Source: CAD feature listing. Evaluate the final solid. Frame: model axes, mm. Face numbers are marked on the shaded views. A direction names the side the tool comes from. Round coordinates to 2 decimals unless told otherwise and drop trailing zeros. Order: outer loops, then holes, each group sorted by start corner. A loop starts at its lowest first (then second) coordinate and runs counter-clockwise, first axis right, second up. Notation, with made-up numbers: (7.25, -30.5) - (50.25, -30.5) arc R7 cw to (50.25, -22.5) - close; hole circle Ø3 at (-35.5, 15). An arc over 180 degrees is marked (long way). Return JSON: item names as keys, results as strings. Group by question number.
1) Section D-D, the plane y = 14. Return loops of the section in (x, z), plus the area to 3 significant figures.
2) Section B-B, the plane y = -11. Return loops of the section in (x, z), plus the area to 3 significant figures.
3) Mould query, pull axis X, two halves, no side actions, for the marked faces 1, 2, 3 and 4. Classes: pulls with the +X half, pulls with the -X half, needs draft (parallel to the pull), parting line crosses it, or undercut.
4) Section C-C, the plane x = 32. Return loops of the section in (y, z), plus the area to 3 significant figures.
5) Access query for the marked faces 5, 6, 7 and 8. Directions: +Z, -Z, +X, -X, +Y, -Y. A direction counts if a zero-diameter tool reaches every point of the face in a straight line with its end or side. Return the directions, or none.
6) Contact query for flat-ended pins moving along their axis: P1, Ø1.5, axis at y = 26.5, z = 3, coming from the +X side; P2, Ø1, axis at y = 24.5, z = 5, coming from the +X side; P3, Ø3, axis at x = 24.5, z = 8, coming from the +Y side. Output: stop coordinate, or through.
7) Ray query, line 1 (Y direction, x = 27, z = 7.5); line 2 (Z direction, x = 22, y = 8.5); line 3 (X direction, y = 14, z = 11.25). Return the intervals inside material, ascending. Write a range as from..to.
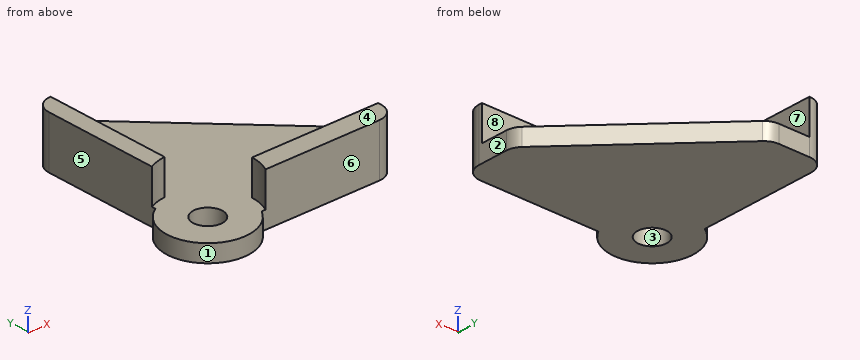
```python
from build123d import *

# Parameters (mm, degrees)
F1_R     = 4.25
F2_DEPTH = 5
F3_DEPTH = 15
F4_R     = 4.99999


# Not quite as in the source:
# - a fillet or chamfer is up to 0.001 mm smaller than in the source, because OpenCascade refuses the exact size
# - a feature names something its author has since deleted; it is built from what else it names


with BuildPart() as f2:
    # F1 (on Top) → F2 (new body)
    with BuildSketch(Plane.XY):
        with BuildLine():
            Line((39.3818591636, 0.8618591636), (-0.6181408364, 0.8618591636))
            Line((-0.6181408364, 0.8618591636), (-0.6181408364, 40.8618591636))
            Line((-0.6181408364, 40.8618591636), (-11.6181408364, 40.8618591636))
            Line((-11.6181408364, 40.8618591636), (-11.6181408364, 3.8233405604))
            ThreePointArc((-11.6181408364, 3.8233405604), (-14.1903183566, 3.3614410672), (-16.6181408364, 2.3944217582))
            Line((-16.6181408364, 2.3944217582), (-16.6181408364, 1.254164009))
            ThreePointArc((-16.6181408364, 1.254164009), (-19.1034222107, -17.6234222107), (-0.225835991, -15.1381408364))
            Line((-0.225835991, -15.1381408364), (0.9144217582, -15.1381408364))
            ThreePointArc((0.9144217582, -15.1381408364), (2.0096719934, -12.2265616521), (2.3818591636, -9.1381408364))
            Line((2.3818591636, -9.1381408364), (39.3818591636, -9.1381408364))
            Line((39.3818591636, -9.1381408364), (39.3818591636, 0.8618591636))
        make_face()
        with Locations((-10.6181408364, -9.1381408364)):
            Circle(F1_R, mode=Mode.SUBTRACT)
        Polygon((-0.6181408364, 40.8618591636), (-0.6181408364, 0.8618591636), (39.3818591636, 0.8618591636), align=None)
    extrude(amount=F2_DEPTH)

    # F1 (on Top) → F3 (join)
    with BuildSketch(Plane.XY):
        with BuildLine():
            Line((39.3818591636, -15.1381408364), (39.3818591636, -9.1381408364))
            Line((39.3818591636, -9.1381408364), (2.3818591636, -9.1381408364))
            ThreePointArc((2.3818591636, -9.1381408364), (2.0096719934, -12.2265616521), (0.9144217582, -15.1381408364))
            Line((0.9144217582, -15.1381408364), (39.3818591636, -15.1381408364))
        make_face()
        with BuildLine():
            Line((-11.6181408364, 3.8233405604), (-11.6181408364, 40.8618591636))
            Line((-11.6181408364, 40.8618591636), (-16.6181408364, 40.8618591636))
            Line((-16.6181408364, 40.8618591636), (-16.6181408364, 2.3944217582))
            ThreePointArc((-16.6181408364, 2.3944217582), (-14.1903183566, 3.3614410672), (-11.6181408364, 3.8233405604))
        make_face()
    extrude(amount=F3_DEPTH)

    # F4 (radius 5 in the source; OpenCascade refuses exactly that, so slightly less here)
    f4_edges = [f2.edges().sort_by_distance(p)[0] for p in [
        (39.381859, -15.138141, 7.5),
        (-16.618141, 40.861859, 7.5),
        (39.381859, 0.861859, 2.5),
        (-0.618141, 40.861859, 2.5),
    ]]
    fillet(f4_edges, radius=F4_R)


solid = f2.part
```
Geometry check:
{
 "1": {"outline": "(-16.62, 0) - (26.24, 0) - (26.24, 5) - (-11.62, 5) - (-11.62, 15) - (-16.62, 15) - close", "area": "264 mm2"},
 "2": {"outline": "(-22.47, 0) - (-14.44, 0) - (-14.44, 5) - (-22.47, 5) - close; (-6.8, 0) - (39.31, 0) - (39.31, 15) - (2.25, 15) - (2.25, 5) - (-6.8, 5) - close", "area": "641 mm2"},
 "3": {"face 1": "parting line crosses it", "face 2": "pulls with the +X half", "face 3": "undercut", "face 4": "needs draft"},
 "4": {"outline": "(-15.14, 0) - (8.24, 0) - (8.24, 5) - (-9.14, 5) - (-9.14, 15) - (-15.14, 15) - close", "area": "177 mm2"},
 "5": {"face 5": "+Z, -Z, -X, +Y", "face 6": "+Z, -Z, +X, -Y", "face 7": "+Z, +X, +Y, -Y", "face 8": "+Z, +X, -X, +Y"},
 "6": {"P1": "x = 14.49", "P2": "x = 16.24", "P3": "y = -9.14"},
 "7": {"line 1": "-15.14..-9.14", "line 2": "0..5", "line 3": "-16.62..-11.62"}
}
